Read the model definition and answer for the solid it produces. Units are mm, in the model's axes. A direction names the side the tool comes from. Give positions to 0.01 mm unless a question says otherwise; leave off trailing zeros. Order: outer loops, then holes, each group sorted by start corner. A loop starts at its lowest first (then second) coordinate and runs counter-clockwise, first axis right, second up. Notation, with made-up numbers: (-22, -6.5) -> (22, -6.5) arc R9 cw to (22, 7.5) -> close; hole circle Ø4 at (-17, 0.25). An arc over 180 degrees is marked (long way). Answer as CSV lines item,"result". Start each with the question number.
1) Find section C-C (y = -1.25). State how many separate pieces and enclosed holes the cut face has, and give its area (3 significant figures).
2) Find section A-A (z = -22.86). Determine the outline of the cut face in (x, y).
3) Find section B-B (x = 49). Determine the outline of the cut face in (y, z), and give its area (3 significant figures).
4) The mould has two halves that part along X. Classify faces 3 (the face through (-12.382, -5, -23)), 4 (the face through (20, 0, -17)), 5 (the face through (38.81, -5.01, -0.69)): +X half, -X half, draft (parallel to the pull), parting line (faces both ways), or undercut.
5) Straight lines are drawn through the part: L1, parallel to Z at x = 16.5, y = -4.75; L2, parallel to X at y = -1.75, z = -1; L3, parallel to X at y = -1.5, z = -22.5. For each, find the intervals that lie inside material, in ascending order. Write a range as from..to.
6) Find section D-D (x = 33). Determine the outline of the cut face in (y, z), and give its area (3 significant figures).
7) For faces 1 (the face through (21, -5, -31.75)), 2 (the face through (22, -5, 3.576)), determine the directions among +Z, -Z, +X, -X, +Y, -Y from which every point of the face is accessible in a straight line to the end or side of a thin tool.
8) Flat-ended cylindrical pins translate along their axes: pin 1 Ø5 at (x, z) = (27.264, -8.509) entering from +Y; pin 2 Ø5 at (x, y) = (25, -7.5) entering from +Z. Find the tip coordinate at first contact, or state that the pin passes through.
```python
from build123d import *

# Parameters (mm, degrees)
SKETCH1_R           = 3.96875
SKETCH1_R_2         = 3.175
SKETCH1_R_3         = 5.3
SKETCH1_R_4         = 1.5
BOSS_EXTRUDE1_DEPTH = 10.16


with BuildPart() as part:
    # Sketch1 → Boss-Extrude1 (new body)
    with BuildSketch(Plane(origin=(0, 0, 0), x_dir=(1, 0, 0), z_dir=(0, 1, 0))):
        with BuildLine():
            Line((54.2925, 31.75), (-12.3825, 31.75))
            Line((-12.3825, 31.75), (-12.3825, 13.97))
            Line((-12.3825, 13.97), (-7.9375, 0))
            ThreePointArc((-7.9375, 0), (-1.838169821, -7.721725064), (7.086131612, -3.576401128))
            Line((7.086131612, -3.576401128), (36.662919386, -3.576401128))
            ThreePointArc((36.662919386, -3.576401128), (43.781301432, -6.068008813), (48.26, 0))
            Line((48.26, 0), (54.2925, 13.97))
            Line((54.2925, 13.97), (54.2925, 31.75))
        make_face()
        with Locations(Location((0, 0, 0), (0, 0, 270))):
            Circle(SKETCH1_R, mode=Mode.SUBTRACT)
        with Locations(Location((41.91, 0, 0), (0, 0, 270))):
            Circle(SKETCH1_R_2, mode=Mode.SUBTRACT)
        with Locations(Location((46.355, 22.86, 0), (0, 0, 270))):
            Circle(SKETCH1_R, mode=Mode.SUBTRACT)
        with Locations(Location((-4.445, 22.86, 0), (0, 0, 270))):
            Circle(SKETCH1_R, mode=Mode.SUBTRACT)
        with Locations(Location((16.764, 8.509, 0), (0, 0, 270))):
            Circle(SKETCH1_R_3, mode=Mode.SUBTRACT)
        with Locations(Location((6.264, 8.509, 0), (0, 0, 270))):
            Circle(SKETCH1_R_4, mode=Mode.SUBTRACT)
        with Locations(Location((27.264, 8.509, 0), (0, 0, 270))):
            Circle(SKETCH1_R_4, mode=Mode.SUBTRACT)
    extrude(amount=-BOSS_EXTRUDE1_DEPTH)


solid = part.part
```
Findings below:
1,separate pieces,"1"
1,enclosed holes,"7"
1,area,"2,020 mm²"
2,outline,"(-12.38, -10.16) -> (-8.41, -10.16) -> (-8.41, 0) -> (-12.38, 0) -> close; (-0.48, -10.16) -> (42.39, -10.16) -> (42.39, 0) -> (-0.48, 0) -> close; (50.32, -10.16) -> (54.29, -10.16) -> (54.29, 0) -> (50.32, 0) -> close"
3,outline,"(-10.16, -31.75) -> (0, -31.75) -> (0, -25.82) -> (-10.16, -25.82) -> close; (-10.16, -19.9) -> (0, -19.9) -> (0, -1.71) -> (-10.16, -1.71) -> close"
3,area,"245 mm²"
4,face 3,"-X half"
4,face 4,"draft"
4,face 5,"undercut"
5,L1,"-31.75..-13.8, -3.22..3.58"
5,L2,"-8.26..-3.84, 3.84..38.9, 44.92..48.69"
5,L3,"-12.38..-8.4, -0.49..42.4, 50.31..54.29"
6,outline,"(-10.16, -31.75) -> (0, -31.75) -> (0, 3.58) -> (-10.16, 3.58) -> close"
6,area,"359 mm²"
7,face 1,"-Z, +X, -X, +Y, -Y"
7,face 2,"+Z, +Y, -Y"
8,pin 1,"y = 0"
8,pin 2,"z = 3.58"
